Work out the finished part from the listing and answer in its coordinate system (mm). Round coordinates to 2 decimals unless told otherwise and drop trailing zeros. Loops run counter-clockwise (first coordinate to the right, second up) from the corner with the lowest first, then second, coordinate; pieces in that order, holes last. Notation, with made-up numbers: (14.25, 49) -> (20.25, 49) arc R20 cw to (20.25, 53) -> close; hole circle Ø11 at (-6.75, 8). An arc over 180 degrees is marked (long way). Write item = value, one per line. Start each with the question number.
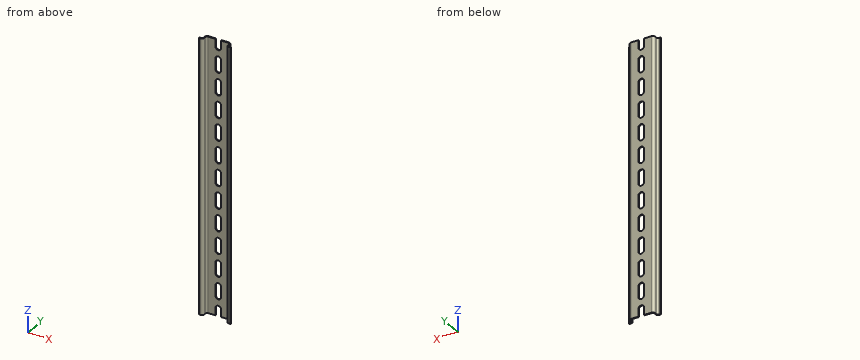
```python
from build123d import *

# Parameters (mm, degrees)
EXTRUDE_MAIN_DEPTH     = 152.5
SLOT_CUT_DEPTH         = 8.5
SLOT_PATTERN_COUNT     = 7
SLOT_PATTERN_PITCH     = 25
SLOT_PATTERN_COL_COUNT = 7
SLOT_PATTERN_COL_PITCH = 25


with BuildPart() as part:
    # Sketch1 → Extrude_main (new body, symmetric)
    with BuildSketch(Plane.XY):
        with BuildLine():
            Line((-17.5, 0), (-15.8, 0))
            ThreePointArc((-15.8, 0), (-13.820101013, 0.820101013), (-13, 2.8))
            Line((-13, 2.8), (-13, 4.7))
            ThreePointArc((-13, 4.7), (-12.472792206, 5.972792206), (-11.2, 6.5))
            Line((-11.2, 6.5), (11.2, 6.5))
            ThreePointArc((11.2, 6.5), (12.472792206, 5.972792206), (13, 4.7))
            Line((13, 4.7), (13, 2.8))
            ThreePointArc((13, 2.8), (13.820101013, 0.820101013), (15.8, 0))
            Line((15.8, 0), (17.5, 0))
            Line((17.5, 0), (17.5, 1))
            Line((17.5, 1), (15.8, 1))
            ThreePointArc((15.8, 1), (14.527207794, 1.527207794), (14, 2.8))
            Line((14, 2.8), (14, 4.7))
            ThreePointArc((14, 4.7), (13.179898987, 6.679898987), (11.2, 7.5))
            Line((11.2, 7.5), (-11.2, 7.5))
            ThreePointArc((-11.2, 7.5), (-13.179898987, 6.679898987), (-14, 4.7))
            Line((-14, 4.7), (-14, 2.8))
            ThreePointArc((-14, 2.8), (-14.527207794, 1.527207794), (-15.8, 1))
            Line((-15.8, 1), (-17.5, 1))
            Line((-17.5, 1), (-17.5, 0))
        make_face()
    extrude(amount=EXTRUDE_MAIN_DEPTH, both=True)

    # Sketch2 → slot_cut (cut, through all)
    with BuildSketch(Plane(origin=(0, 0, 0), x_dir=(1, 0, 0), z_dir=(0, 1, 0))):
        with BuildLine():
            Line((-3.175, 5.825), (-3.175, -5.825))
            ThreePointArc((-3.175, -5.825), (0, -9), (3.175, -5.825))
            Line((3.175, -5.825), (3.175, 5.825))
            ThreePointArc((3.175, 5.825), (0, 9), (-3.175, 5.825))
        make_face()
    slot_cut = extrude(amount=SLOT_CUT_DEPTH, mode=Mode.SUBTRACT)

    # slot_pattern: slot_cut ×7
    with Locations(*[(0, 0, i * SLOT_PATTERN_PITCH) for i in range(1, SLOT_PATTERN_COUNT)]):
        add(slot_cut, mode=Mode.SUBTRACT)

    # slot_pattern col: slot_cut ×7
    with Locations(*[(0, 0, -i * SLOT_PATTERN_COL_PITCH) for i in range(1, SLOT_PATTERN_COL_COUNT)]):
        add(slot_cut, mode=Mode.SUBTRACT)


solid = part.part
```
Item 1: Flat-ended cylindrical pins translate along their axes: pin 1 (3 mm diameter, centred on y = 4.5, z = -71.5, fed in from +X); pin 2 (0.5 mm diameter, centred on y = 7, z = 52.5, fed in from -X); pin 3 (0.8 mm diameter, centred on y = 7, z = 97.5, fed in from +X). Find the tip coordinate at first contact, or state that the pin passes through.
Item 2: Section B-B (x = 0) is taken. Count the separate pieces of the cut face and the enclosed holes in it, then the cut area to 3 significant figures.
Item 3: Find the intervals of material crossed by line 1 along X through (y, z) = (4.5, 8.5); line 2 along X through (y, z) = (2, 77.5); line 3 along Y through (x, z) = (-15.5, -108.5), in increasing order. Write a range as [from, to].
Item 4: Section A-A (z = -72.5) is taken. Determine the outline of the cut face in (x, y) (3 decimals), then the cut area to 3 significant figures.
Worked answers:
q1.pin_1 = 14
q1.pin_2 = -13.11
q1.pin_3 = 13.26
q2.separate_pieces = 12
q2.enclosed_holes = 0
q2.area = 84.0 mm2
q3.line_1 = [-14, -13], [13, 14]
q3.line_2 = [-14.19, -13.12], [13.12, 14.19]
q3.line_3 = [0.02, 1.03]
q4.outline = (-17.5, 0) -> (-15.8, 0) arc R2.8 ccw to (-13, 2.8) -> (-13, 4.7) arc R1.8 cw to (-11.2, 6.5) -> (-3.175, 6.5) -> (-3.175, 7.5) -> (-11.2, 7.5) arc R2.8 ccw to (-14, 4.7) -> (-14, 2.8) arc R1.8 cw to (-15.8, 1) -> (-17.5, 1) -> close; (3.175, 6.5) -> (11.2, 6.5) arc R1.8 cw to (13, 4.7) -> (13, 2.8) arc R2.8 ccw to (15.8, 0) -> (17.5, 0) -> (17.5, 1) -> (15.8, 1) arc R1.8 cw to (14, 2.8) -> (14, 4.7) arc R2.8 ccw to (11.2, 7.5) -> (3.175, 7.5) -> close
q4.area = 37.7 mm2
